Input: part model. Units: mm. Frame: model coordinates. Face numbers are marked on the shaded views. A direction names the side the tool comes from. Round coordinates to 2 decimals unless told otherwise and drop trailing zeros. Order: outer loops, then holes, each group sorted by start corner. A loop starts at its lowest first (then second) coordinate and runs counter-clockwise, first axis right, second up. Notation, with made-up numbers: M 85,-36.75 L 104,-36.75 A31 cw 104,-1.75 Z; hole C -29,82.5 d7. An arc over 180 degrees is marked long. One line per question, with ' | ' between items.
```python
from build123d import *

# Parameters (mm, degrees)
BOSS_EXTRUDE1_DEPTH = 120
SHELL1_T            = -10
SKETCH2_R           = 29
SKETCH2_R_2         = 1.54318701
CUT_EXTRUDE1_DEPTH  = 200
SKETCH3_W           = 15
SKETCH3_H           = 6.085201518
CUT_EXTRUDE2_DEPTH  = 200
SKETCH4_W           = 32
SKETCH4_H           = 24.066005235
BOSS_EXTRUDE2_DEPTH = 6


with BuildPart() as part:
    # Sketch1 → Boss-Extrude1 (new body)
    with BuildSketch(Plane.XY):
        with BuildLine():
            Line((-10.096774194, 144.410679099), (89.903225806, 144.410679099))
            ThreePointArc((89.903225806, 144.410679099), (126.330854691, 69.550051356), (139.903225806, -12.589320901))
            Line((139.903225806, -12.589320901), (-10.096774194, -12.589320901))
            Line((-10.096774194, -12.589320901), (-10.096774194, 144.410679099))
        make_face()
    extrude(amount=BOSS_EXTRUDE1_DEPTH)

    # Shell1
    shell1_openings = [part.faces().sort_by_distance(p)[0] for p in [
        (120.617040249, 67.730365228, 60),
    ]]
    offset(amount=SHELL1_T, openings=shell1_openings, kind=Kind.INTERSECTION)

    # Sketch2 → Cut-Extrude1 (cut)
    with BuildSketch(Plane.XY.offset(120)):
        with Locations((39.903225806, 90.410679099)):
            Circle(SKETCH2_R)
        with Locations((79.903225806, 137.910679099)):
            Circle(SKETCH2_R_2)
        with Locations((64.903225806, 137.910679099)):
            Circle(SKETCH2_R_2)
    extrude(amount=-CUT_EXTRUDE1_DEPTH, mode=Mode.SUBTRACT)

    # Sketch3 → Cut-Extrude2 (cut)
    with BuildSketch(Plane.XY.offset(120)):
        Polygon((75.215541826, -12.589320901), (81.300743344, -6.504119383), (83.903225806, -6.504119383), (89.988427324, -12.589320901), align=None)
        with Locations((17.715541826, -9.546720142)):
            Rectangle(SKETCH3_W, SKETCH3_H)
    extrude(amount=-CUT_EXTRUDE2_DEPTH, mode=Mode.SUBTRACT)

    # Sketch4 → Boss-Extrude2 (add)
    with BuildSketch(Plane.XY.offset(120)):
        with Locations((5.903225806, 132.377676482)):
            Rectangle(SKETCH4_W, SKETCH4_H)
    extrude(amount=BOSS_EXTRUDE2_DEPTH)


solid = part.part
```
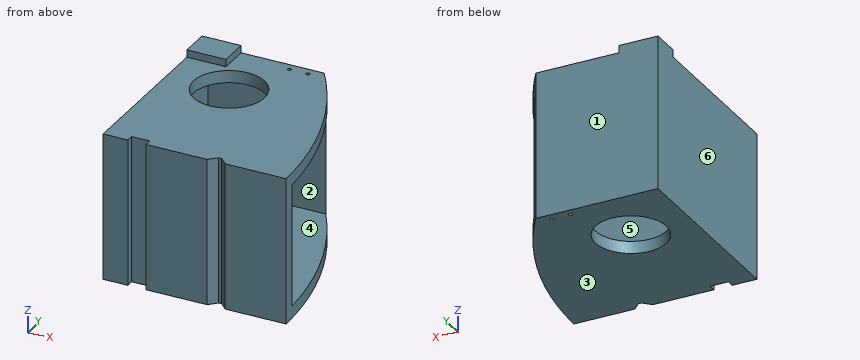
Item 1: Mould query, pull axis Z, two halves, no side actions, for the marked faces 3, 4, 5 and 6. Classes: +Z half, -Z half, draft (parallel to the pull), parting line (faces both ways), or undercut.
Report:
face 3: -Z half | face 4: undercut | face 5: undercut | face 6: draft
Item 2: Section query B-B, the plane x = 127. Return loops of the section in (y, z).
Report:
outline: M -12.59,0 L 67.42,0 L 67.42,10 L -2.59,10 L -2.59,110 L 67.42,110 L 67.42,120 L -12.59,120 Z
Item 3: Section query C-C, the plane z = 43. Return loops of the section in (x, y).
Report:
outline: M -10.1,-12.59 L 10.22,-12.59 L 10.22,-6.5 L 25.22,-6.5 L 25.22,-12.59 L 75.22,-12.59 L 81.3,-6.5 L 83.9,-6.5 L 89.99,-12.59 L 139.9,-12.59 A288.96 ccw 139.54,-2.59 L -0.1,-2.59 L -0.1,134.41 L 96.41,134.41 A288.96 ccw 89.9,144.41 L -10.1,144.41 Z; hole C 64.9,137.91 d3.09; hole C 79.9,137.91 d3.09
Item 4: First-contact query: pin 1 (1 mm diameter, centred on x = 96.5, z = 71.5, fed in from +Y); pin 2 (3 mm diameter, centred on x = 3.5, z = 124.5, fed in from -Y); pin 3 (4 mm diameter, centred on x = 64.9, y = 137.91, fed in from -Z); pin 4 (4.5 mm diameter, centred on x = 17, z = 67.5, fed in from -Y). Flat tips, straight axial feed; report the tip coordinate or a pass-through.
Report:
pin 1: y = 135.07 | pin 2: y = 120.34 | pin 3: z = 0 | pin 4: y = -6.5
Item 5: Access query for the marked faces 1 and 2. Directions: +Z, -Z, +X, -X, +Y, -Y. A direction counts if a zero-diameter tool reaches every point of the face in a straight line with its end or side. Return the directions, or none.
Report:
face 1: +Z, -Z, +X, -X, +Y | face 2: +X
Item 6: Section query A-A, the plane y = 74. Return loops of the section in (x, z), plus the area to 3 significant figures.
Report:
outline: M -10.1,0 L 15.99,0 L 15.99,10 L -0.1,10 L -0.1,110 L 15.99,110 L 15.99,120 L -10.1,120 Z; M 63.81,0 L 124.87,0 L 124.87,10 L 63.81,10 Z; M 63.81,110 L 124.87,110 L 124.87,120 L 63.81,120 Z | area: 2,740 mm²
Item 7: Section query D-D, the plane y = 128.5. Return loops of the section in (x, z), plus the area to 3 significant figures.
Report:
outline: M -10.1,0 L 99.99,0 L 99.99,10 L -0.1,10 L -0.1,110 L 99.99,110 L 99.99,120 L 21.9,120 L 21.9,126 L -10.1,126 Z | area: 3,390 mm²
Item 8: Line query: line 1 along Y through (x, z) = (38, 52.5); line 2 along Z through (x, y) = (35, 6); line 3 along X through (y, z) = (137.5, 93.5). Output: solid intervals per line, ascending. Write a range as from..to.
Report:
line 1: -12.59..-2.59, 134.41..144.41 | line 2: 0..10, 110..120 | line 3: -10.1..63.42, 66.39..78.42, 81.39..94.46
